For this review, take the finished solid that the model builds, in its own axes (mm). Face numbers are marked on the shaded views. Coordinates: 2 decimals unless noted, no trailing zeros. Write each loop counter-clockwise with the first axis right and the second up, starting at its lowest first coordinate (ties: lowest second). Pieces come first, ordered by that corner, then holes. Notation, with made-up numbers: M -38.5,57.5 L -11.5,57.5 A22 ccw -11.5,80.5 Z; hole C -25.5,65.5 d6. An arc over 180 degrees is marked long. Return JSON: item names as keys, results as strings.
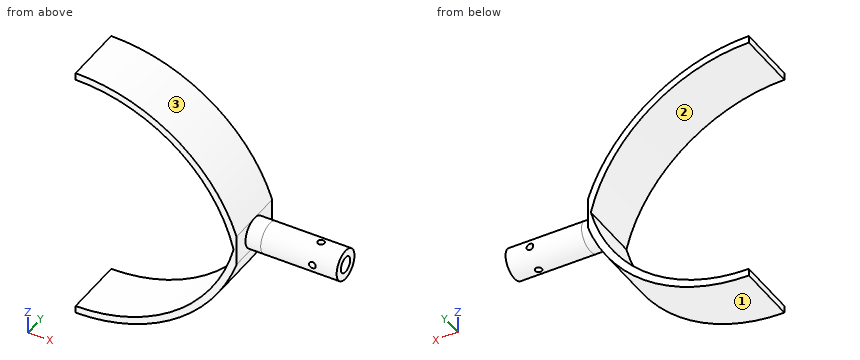
```python
from build123d import *

# Parameters (mm, degrees)
SKETCH1_R                = 5
BOSS_EXTRUDE1_DEPTH      = 25
SKETCH2_R                = 2.6
CUT_EXTRUDE1_DEPTH       = 25
CUT_EXTRUDE3_DEPTH       = 25
CUT_EXTRUDE3_DEPTH_BACK  = 25
SKETCH3_R                = 1.1
CUT_EXTRUDE4_DEPTH       = 25
CUT_EXTRUDE4_DEPTH_BACK  = 25
SKETCH4_R                = 1.1
BOSS_EXTRUDE3_START      = 5
SKETCH6_R                = 5
BOSS_EXTRUDE3_DEPTH      = 5
BOSS_EXTRUDE2_DEPTH      = 10
BOSS_EXTRUDE2_DEPTH_BACK = 10


with BuildPart() as part:
    # Sketch1 → Boss-Extrude1 (new body)
    with BuildSketch(Plane(origin=(0, 0, 0), x_dir=(0, 0, -1), z_dir=(1, 0, 0))):
        Circle(SKETCH1_R)
    extrude(amount=BOSS_EXTRUDE1_DEPTH)

    # Sketch2 → Cut-Extrude1 (cut)
    with BuildSketch(Plane.ZY):
        Circle(SKETCH2_R)
    extrude(amount=-CUT_EXTRUDE1_DEPTH, mode=Mode.SUBTRACT)

    # Sketch3 → Cut-Extrude3 (cut, two sides: drawn at the far end of the back side and taken through both)
    with BuildSketch(Plane(origin=(0, 0, 0), x_dir=(1, 0, 0), z_dir=(0, 1, 0)).offset(-CUT_EXTRUDE3_DEPTH_BACK)):
        with Locations(Location((17, 0, 0), (0, 0, 90))):
            Circle(SKETCH3_R)
    extrude(amount=CUT_EXTRUDE3_DEPTH + CUT_EXTRUDE3_DEPTH_BACK, mode=Mode.SUBTRACT)

    # Sketch4 → Cut-Extrude4 (cut, two sides: drawn at the far end of the back side and taken through both)
    with BuildSketch(Plane.XY.offset(-CUT_EXTRUDE4_DEPTH_BACK)):
        with Locations(Location((17, 0, 0), (0, 0, 180))):
            Circle(SKETCH4_R)
    extrude(amount=CUT_EXTRUDE4_DEPTH + CUT_EXTRUDE4_DEPTH_BACK, mode=Mode.SUBTRACT)

    # Sketch6 → Boss-Extrude3 (add)
    with BuildSketch(Plane.ZY.offset(BOSS_EXTRUDE3_START)):
        Circle(SKETCH6_R)
    extrude(amount=-BOSS_EXTRUDE3_DEPTH)

    # Sketch5 → Boss-Extrude2 (add, two sides: drawn at the far end of the back side and taken through both)
    with BuildSketch(Plane(origin=(0, 0, 0), x_dir=(1, 0, 0), z_dir=(0, 1, 0)).offset(-BOSS_EXTRUDE2_DEPTH_BACK)):
        with BuildLine():
            ThreePointArc((-58, 40.633969476), (-25.001840156, 29.270877002), (-5.996204592, 0))
            ThreePointArc((-5.996204592, 0), (-5.43861434, 2.488147565), (-5, 5))
            ThreePointArc((-5, 5), (-25.392485529, 32.518375447), (-58, 43))
            Line((-58, 43), (-58, 40.633969476))
        make_face()
        with BuildLine():
            Line((-58, -40.633969476), (-58, -43))
            ThreePointArc((-58, -43), (-25.392485529, -32.518375447), (-5, -5))
            ThreePointArc((-5, -5), (-5.43861434, -2.488147565), (-5.996204592, 0))
            ThreePointArc((-5.996204592, 0), (-25.001840156, -29.270877002), (-58, -40.633969476))
        make_face()
        with BuildLine():
            ThreePointArc((-5.996204592, 0), (-5.43861434, -2.488147565), (-5, -5))
            Line((-5, -5), (-5, 5))
            ThreePointArc((-5, 5), (-5.43861434, 2.488147565), (-5.996204592, 0))
        make_face()
    extrude(amount=BOSS_EXTRUDE2_DEPTH + BOSS_EXTRUDE2_DEPTH_BACK)


solid = part.part
```
1. Draft analysis for pull direction Z (two halves, no side actions). For the marked faces 1, 2 and 3, state which applies: +Z half, -Z half, draft (parallel to the pull), parting line (faces both ways), or undercut.
Checks:
{"face 1": "-Z half", "face 2": "undercut", "face 3": "+Z half"}
2. Clearance check with flat-ended pins moving along their axes: pin 1 Ø2 at (y, z) = (7.5, 26) entering from +X; pin 2 Ø3.5 at (x, z) = (17, 0) entering from -Y; pin 3 Ø3 at (x, z) = (17, 0) entering from +Y; pin 4 Ø5 at (y, z) = (-6.5, -2) entering from +X. State where each tip first meets the part, or that it passes through.
Checks:
{"pin 1": "x = -16.88", "pin 2": "y = -5", "pin 3": "y = 5", "pin 4": "x = 25"}
3. We need section B-B (x = 17). State the section outline as (y, z) points, plus the area to 3 significant figures.
Checks:
{"outline": "M -4.88,-1.1 A5 ccw -1.1,-4.88 L -1.1,-2.36 A2.6 cw -2.36,-1.1 Z; M -4.88,1.1 L -2.36,1.1 A2.6 cw -1.1,2.36 L -1.1,4.88 A5 ccw Z; M 1.1,-4.88 A5 ccw 4.88,-1.1 L 2.36,-1.1 A2.6 cw 1.1,-2.36 Z; M 1.1,2.36 A2.6 cw 2.36,1.1 L 4.88,1.1 A5 ccw 1.1,4.88 Z", "area": "35.8 mm2"}
4. We need section A-A (x = -10). State the section outline as (y, z) points, plus the area to 3 significant figures.
Checks:
{"outline": "M -10,-15.81 L 10,-15.81 L 10,-10.88 L -10,-10.88 Z; M -10,10.88 L 10,10.88 L 10,15.81 L -10,15.81 Z", "area": "197 mm2"}
5. Wall thickness on L1, parallel to Y at x = 10.75, z = 0; L2, parallel to Z at x = -26.5, y = -6.5; L3, parallel to Z at x = 17, y = 4.3: over which ranges is each line inside the solid? List them lowest first. Write a range as from..to.
Checks:
{"L1": "-5..-2.6, 2.6..5", "L2": "-33.29..-30.4, 30.4..33.29", "L3": "-2.55..-1.1, 1.1..2.55"}
6. We need section C-C (y = 8). State the section outline as (x, z) points, plus the area to 3 significant figures.
Checks:
{"outline": "M -58,-43 A55.96 ccw -5,-5 L -5,5 A55.96 ccw -58,43 L -58,40.63 A53.59 cw -6,0 A53.59 cw -58,-40.63 Z", "area": "338 mm2"}
7. We need section D-D (x = 8). State the section outline as (y, z) points, plus the area to 3 significant figures.
Checks:
{"outline": "C 0,0 d10; hole C 0,0 d5.2", "area": "57.3 mm2"}
